Geometry check sheet. Reference: drawing and pictorial views, mm from the part's lowest x, y, z. A direction names the side the tool comes from. Give positions to 0.01 mm unless a question says otherwise; leave off trailing zeros. Order: outer loops, then holes, each group sorted by start corner. A loop starts at its lowest first (then second) coordinate and runs counter-clockwise, first axis right, second up.
Item 1: Sectioned sample at C-C on x = 268. Record the boundary of the cut face in (y, z), and give its area (3 significant figures).
Item 2: Material ranges on line 1 along X through (y, z) = (187.5, 18); line 2 along Y through (x, z) = (55.5, 32); line 3 along Z through (x, y) = (301.5, 211), recorded low to high.
Item 3: Release check for a two-part mould opening along X. For the marked faces 1, 2 and 3 record: released by +X, released by -X, zero draft, split by the parting line, or undercut.
Item 4: Sectioned sample at A-A on z = 16. Record the boundary of the cut face in (x, y).
Item 5: Sectioned sample at B-B on y = 186. Record the boundary of the cut face in (x, z), and give its area (3 significant figures).
Item 6: Access from +Z, -Z, +X, -X, +Y, -Y to the whole of each face (thin tool, end or side, straight path). Record for the marked faces 4 and 5.
Item 7: Gauge pin test, flat ends, axial feed: P1, Ø10, axis at x = 82, z = 15, coming from the -Y side; P2, Ø24, axis at x = 73, y = 161.5, coming from the -Z side. Record the tip position at first contact, or that the pin passes through.
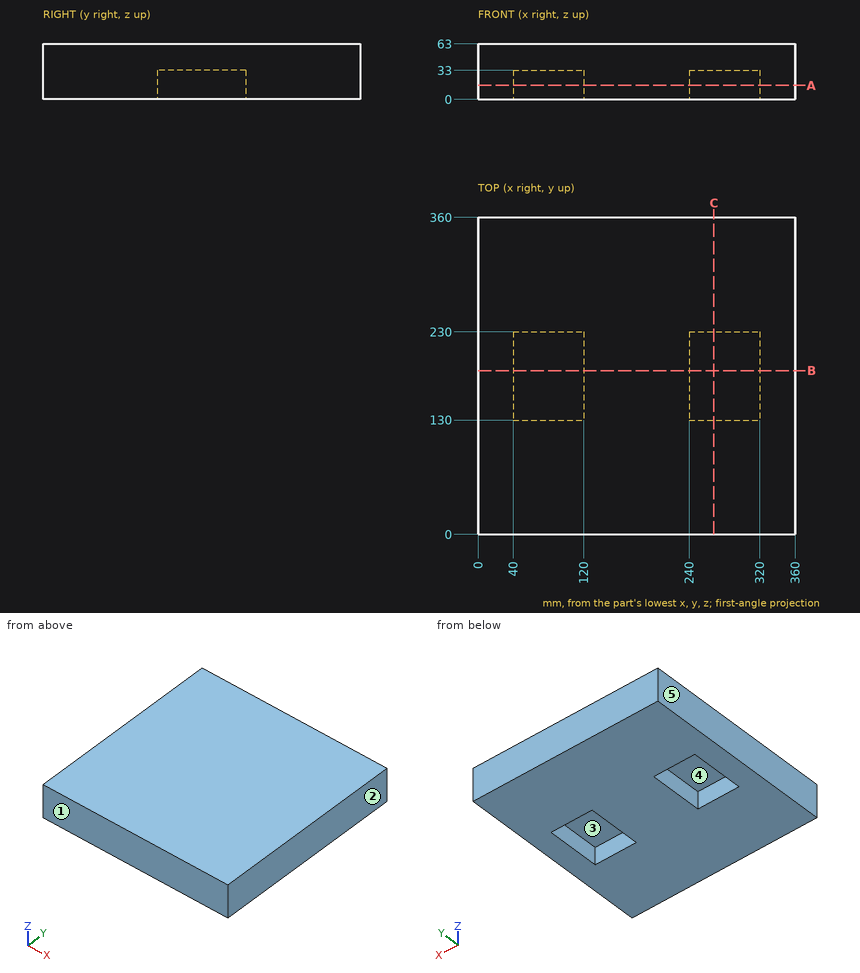
Report:
1. outline: (0, 0) - (130, 0) - (130, 33) - (230, 33) - (230, 0) - (360, 0) - (360, 63) - (0, 63) - close
1. area: 19,400 mm2
2. line 1: x = 0 to 40, 120 to 240, 320 to 360
2. line 2: y = 0 to 130, 230 to 360
2. line 3: z = 33 to 63
3. face 1: zero draft
3. face 2: released by +X
3. face 3: undercut
4. outline: (0, 0) - (360, 0) - (360, 360) - (0, 360) - close; hole (40, 130) - (120, 130) - (120, 230) - (40, 230) - close; hole (240, 130) - (320, 130) - (320, 230) - (240, 230) - close
5. outline: (0, 0) - (40, 0) - (40, 33) - (120, 33) - (120, 0) - (240, 0) - (240, 33) - (320, 33) - (320, 0) - (360, 0) - (360, 63) - (0, 63) - close
5. area: 17,400 mm2
6. face 4: -Z
6. face 5: +Z, -Z, -X, +Y, -Y
7. P1: stops at y = 0
7. P2: stops at z = 33
